from build123d import *

# Parameters (mm, degrees)
EXTRUDE_1_DEPTH      = 8
EXTRUDE_2_DEPTH      = 10
SKETCH_1_5_W         = 100
SKETCH_1_5_H         = 16
EXTRUDE_3_DEPTH      = 42
EXTRUDE_START        = 12
SKETCH_1_6_W         = 100
SKETCH_1_6_H         = 4
EXTRUDE_4_DEPTH      = 18
SKETCH_2_R           = 3.5
CUT_EXTRUDE_4_DEPTH  = 123.995934892
EXTRUDE_7_DEPTH      = 8
EXTRUDE_8_DEPTH      = 20
EXTRUDE_8_DEPTH_BACK = 10
RIB_START            = -3.5
RIB_2_DEPTH          = 7


# Read off the part's stored shape, not the designer's step: 筋2
with BuildPart() as part:
    # 草图1 → 凸台-拉伸1 (new body)
    with BuildSketch(Plane(origin=(0, 0, 0), x_dir=(0, 0, -1), z_dir=(1, 0, 0))):
        with BuildLine():
            Line((2.152816021, 55.078639964), (-50, 10))
            Line((-50, 10), (50, 10))
            Line((50, 10), (50, 46))
            ThreePointArc((50, 46), (46.485281374, 37.514718626), (38, 34))
            Line((38, 34), (10, 34))
            ThreePointArc((10, 34), (-1.245969935, 41.813335431), (2.152816021, 55.078639964))
        make_face()
    extrude(amount=EXTRUDE_1_DEPTH)

    # 草图1<3> → 凸台-拉伸2 (add)
    with BuildSketch(Plane(origin=(0, 0, 0), x_dir=(0, 0, -1), z_dir=(1, 0, 0))):
        with BuildLine():
            ThreePointArc((38, 34), (50, 46), (38, 58))
            Line((38, 58), (10, 58))
            ThreePointArc((10, 58), (-2, 46), (10, 34))
            Line((10, 34), (38, 34))
        make_face()
        with BuildLine():
            ThreePointArc((38, 40), (44, 46), (38, 52))
            Line((38, 52), (10, 52))
            ThreePointArc((10, 52), (4, 46), (10, 40))
            Line((10, 40), (38, 40))
        make_face(mode=Mode.SUBTRACT)
    extrude(amount=EXTRUDE_2_DEPTH)

    # 草图1<5> → 凸台-拉伸3 (add)
    with BuildSketch(Plane(origin=(0, 0, 0), x_dir=(0, 0, -1), z_dir=(1, 0, 0))):
        with Locations((0, 2)):
            Rectangle(SKETCH_1_5_W, SKETCH_1_5_H)
    extrude(amount=EXTRUDE_3_DEPTH)

    # 草图1<6> → 凸台-拉伸4 (add)
    with BuildSketch(Plane(origin=(0, 0, 0), x_dir=(0, 0, -1), z_dir=(1, 0, 0)).offset(EXTRUDE_START)):
        with Locations((0, -8)):
            Rectangle(SKETCH_1_6_W, SKETCH_1_6_H)
    extrude(amount=EXTRUDE_4_DEPTH)

    # 草图2 → 切除-拉伸4 (cut, through all)
    with BuildSketch(Plane.XY.offset(50)):
        with Locations((21, 3)):
            Circle(SKETCH_2_R)
    extrude(amount=-CUT_EXTRUDE_4_DEPTH, mode=Mode.SUBTRACT)

    # 草图4 → 凸台-拉伸7 (add)
    with BuildSketch(Plane(origin=(0, 10, 0), x_dir=(1, 0, 0), z_dir=(0, 1, 0))):
        with BuildLine():
            ThreePointArc((54, 0), (60.846702456, 10.837136357), (73.573920737, 9.307831362))
            Line((73.573920737, 9.307831362), (42, 35))
            Line((42, 35), (42, 0))
            Line((42, 0), (54, 0))
        make_face()
        with BuildLine():
            Line((42, -35), (73.573920737, -9.307831362))
            ThreePointArc((73.573920737, -9.307831362), (60.846702456, -10.837136357), (54, 0))
            Line((54, 0), (42, 0))
            Line((42, 0), (42, -35))
        make_face()
    extrude(amount=-EXTRUDE_7_DEPTH)

    # 草图4<3> → 凸台-拉伸8 (add, two sides: drawn at the far end of the back side and taken through both)
    with BuildSketch(Plane(origin=(0, 10, 0), x_dir=(1, 0, 0), z_dir=(0, 1, 0)).offset(-EXTRUDE_8_DEPTH_BACK)):
        with BuildLine():
            ThreePointArc((60, 0), (66, 6), (72, 0))
            Line((72, 0), (78, 0))
            ThreePointArc((78, 0), (76.837136357, 5.153297544), (73.573920737, 9.307831362))
            ThreePointArc((73.573920737, 9.307831362), (60.846702456, 10.837136357), (54, 0))
            Line((54, 0), (60, 0))
        make_face()
        with BuildLine():
            Line((78, 0), (72, 0))
            ThreePointArc((72, 0), (66, -6), (60, 0))
            Line((60, 0), (54, 0))
            ThreePointArc((54, 0), (60.846702456, -10.837136357), (73.573920737, -9.307831362))
            ThreePointArc((73.573920737, -9.307831362), (76.837136357, -5.153297544), (78, 0))
        make_face()
    extrude(amount=EXTRUDE_8_DEPTH + EXTRUDE_8_DEPTH_BACK)

    # 筋2 outline → 筋2 (add)
    with BuildSketch(Plane.XY.offset(RIB_START)):
        Polygon((56, 27), (52, 27), (42, 10), (56, 10), align=None)
    extrude(amount=RIB_2_DEPTH)


solid = part.part
For this review, take the finished solid that the model builds, in its own axes (mm). A direction names the side the tool comes from. Round coordinates to 2 decimals unless told otherwise and drop trailing zeros. Order: outer loops, then holes, each group sorted by start corner. A loop starts at its lowest first (then second) coordinate and runs counter-clockwise, first axis right, second up. Notation, with made-up numbers: M 37.5,-35.5 L 77.5,-35.5 A12 cw 77.5,-28.5 Z; hole C 11,-31 d11. An arc over 180 degrees is marked long. Use a Markdown table: item, result. Add a question column.
Item 1: Tool access review of faces 4 (the flat face through (10, 54, -24)), 5 (the flat face through (30, -8, 1)), 6 (the cylindrical face through (5, 46, -4)), 7 (the flat face through (12, -8, 1)): name each direction out of +Z, -Z, +X, -X, +Y, -Y from which nothing blocks a thin tool from reaching the whole face with its end or side.
Item 2: Add section D-D, the plane y = 49. Give the boundary of the cut face in (x, z), then the cut area to 3 significant figures.
Item 3: To check wall thickness, follow line 1 along Z through (x, y) = (66, 23); line 2 along X through (y, z) = (21.25, 0); line 3 along Y through (x, z) = (56.5, 7.5). State the ranges of each line that lie inside material, in increasing order.
Item 4: Mouldability with a two-part tool opening along Z and no side actions: class faces 1 (the cylindrical face through (6.04, 53.51, -47.36)), 2 (the cylindrical face through (5, 46, -44)), 3 (the flat face through (51, 2, 0)) as released by +Z, released by -Z, zero draft, split by the parting line, or undercut.
Item 5: Add section C-C, the plane x = 21. Give the boundary of the cut face in (y, z).
Item 6: Add section A-A, the plane y = 16. Give the boundary of the cut face in (x, z).
Item 7: Add section B-B, the plane z = -25. Give the boundary of the cut face in (x, y).
Item 8: Insertion check: pin 1 (13.5 mm diameter, centred on y = 24.5, z = 19, fed in from +X); pin 2 (10 mm diameter, centred on x = 62, z = -6, fed in from -Y); pin 3 (1 mm diameter, centred on y = 5.5, z = -24, fed in from +X). Each pin has a flat end and moves straight along its axis. Give the tip position at first contact, or say it passes through.
Geometry results:
| question | item | result |
|---|---|---|
| 1 | face 4 | +Z, -Z, +X, +Y |
| 1 | face 5 | +Z, -Z, +X, -Y |
| 1 | face 6 | +X, -X |
| 1 | face 7 | +Z, -Z, -X, -Y |
| 2 | outline | M 0,-49.62 L 10,-49.62 L 10,-43.2 L 0,-43.2 Z; M 0,-4.8 L 10,-4.8 L 10,1.62 L 8,1.62 L 8,4.88 L 0,4.88 Z |
| 2 | area | 155 mm² |
| 3 | line 1 | z = -12 to -6, 6 to 12 |
| 3 | line 2 | x = 0 to 8, 48.62 to 60, 72 to 78 |
| 3 | line 3 | y = 2 to 10 |
| 4 | face 1 | released by -Z |
| 4 | face 2 | undercut |
| 4 | face 3 | zero draft |
| 5 | outline | M -10,-50 L -0.5,-50 L -0.5,50 L -10,50 Z; M 6.5,-50 L 10,-50 L 10,50 L 6.5,50 Z |
| 6 | outline | M 0,-50 L 8,-50 L 8,43.06 L 0,43.06 Z; M 45.53,-3.5 L 54.52,-3.5 A12 ccw long 54.52,3.5 L 45.53,3.5 Z; hole C 66,0 d12 |
| 7 | outline | M 0,-6 L 12,-6 L 12,-10 L 30,-10 L 30,-6 L 42,-6 L 42,2 L 54.29,2 L 54.29,10 L 8,10 L 8,34 L 10,34 L 10,40 L 0,40 Z; M 0,52 L 10,52 L 10,58 L 0,58 Z; hole C 21,3 d7 |
| 8 | pin 1 | stops at x = 8 |
| 8 | pin 2 | stops at y = 0 |
| 8 | pin 3 | stops at x = 56.13 |
